Here's the drawing with two shaded views (mm, measured from the low corner). I have some questions. A direction names the side the tool comes from. Coordinates: 2 decimals unless noted, no trailing zeros. Order: outer loops, then holes, each group sorted by start corner. A loop starts at its lowest first (then second) coordinate and runs counter-clockwise, first axis right, second up. Notation, with made-up numbers: (30.25, 9) - (88.25, 9) arc R25 cw to (88.25, 46) - close; hole circle Ø3 at (48, 85). An arc over 180 degrees is marked (long way). Answer as CSV lines item,"result". Start each with the question number.
1. I want a section at C-C, the plane x = 128.5. List the corners of the cut face in (y, z) for me, and give its area (3 significant figures).
2. I want a section at B-B, the plane y = 5. List the corners of the cut face in (x, z) for me.
3. I want a section at D-D, the plane y = 23. List the corners of the cut face in (x, z) for me.
4. I want a section at A-A, the plane x = 85. List the corners of the cut face in (y, z) for me, and give its area (3 significant figures).
5. For the marked faces 1 and 2, which set-ups out of +Z, -Z, +X, -X, +Y, -Y let a thin tool reach every point of the face, with its end or its side?
6. I need wall thicknesses on probe 1 along Y at (x, z) = (85, 79.2); probe 2 along Y at (x, z) = (37, 16); probe 3 along Z at (x, y) = (84.5, 22). Which ranges of each line are inside material? Lowest first, please.
7. For pin 1 (0.6 mm diameter, centred on y = 13.5, z = 79, fed in from -X); pin 2 (5 mm diameter, centred on x = 28, z = 33.5, fed in from -Y); pin 3 (4 mm diameter, centred on x = 31, y = 34.5, fed in from -Z); pin 4 (1.5 mm diameter, centred on x = 90, y = 8.5, fed in from -Z), each with a flat end and sliding along its axis, tell me the tip position at first contact or that it passes through.
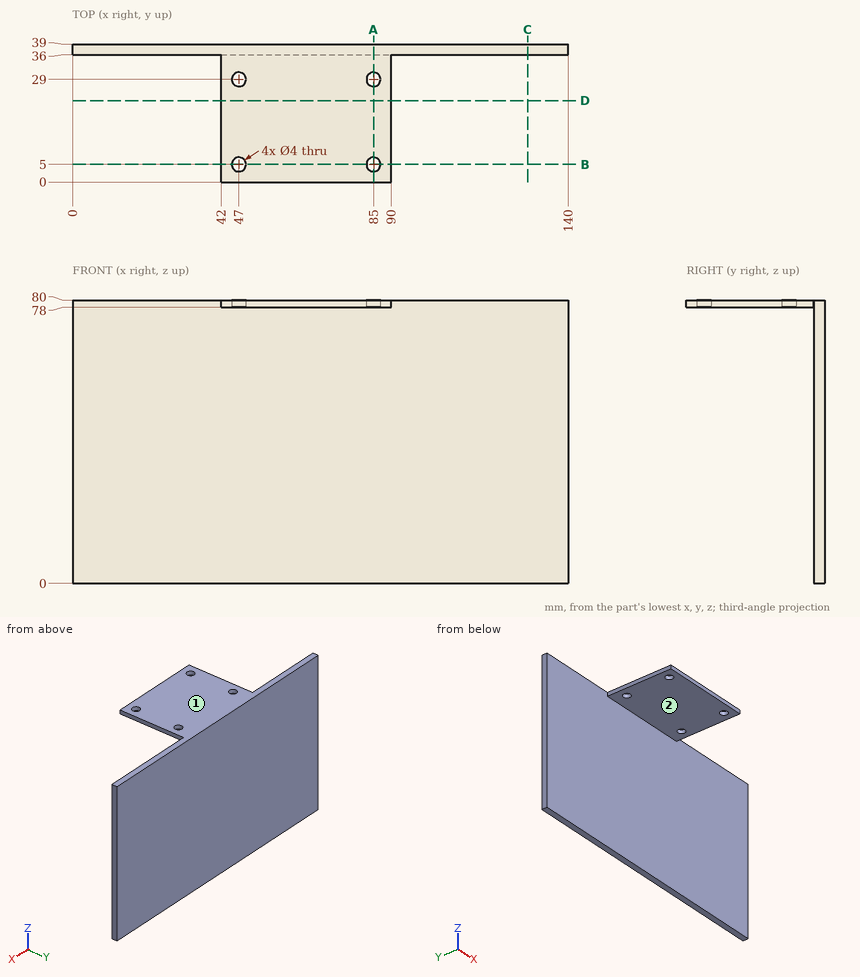
Solved:
1,outline,"(36, 0) - (39, 0) - (39, 80) - (36, 80) - close"
1,area,"240 mm2"
2,outline,"(42, 78) - (45, 78) - (45, 80) - (42, 80) - close; (49, 78) - (83, 78) - (83, 80) - (49, 80) - close; (87, 78) - (90, 78) - (90, 80) - (87, 80) - close"
3,outline,"(42, 78) - (90, 78) - (90, 80) - (42, 80) - close"
4,outline,"(0, 78) - (3, 78) - (3, 80) - (0, 80) - close; (7, 78) - (27, 78) - (27, 80) - (7, 80) - close; (31, 78) - (36, 78) - (36, 0) - (39, 0) - (39, 80) - (31, 80) - close"
4,area,"296 mm2"
5,face 1,"+Z, +X, -X, +Y, -Y"
5,face 2,"-Z, +X, -X, -Y"
6,probe 1,"y = 0 to 3, 7 to 27, 31 to 39"
6,probe 2,"y = 36 to 39"
6,probe 3,"z = 78 to 80"
7,pin 1,"stops at x = 42"
7,pin 2,"stops at y = 36"
7,pin 3,"stops at z = 0"
7,pin 4,"stops at z = 78"
